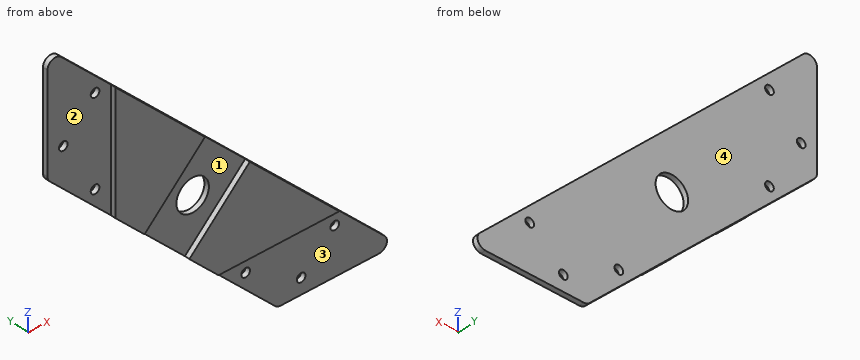
```python
from build123d import *

# Parameters (mm, degrees)
SKETCH1_R           = 10.25
BOSS_EXTRUDE1_DEPTH = 3.175
BOSS_EXTRUDE2_DEPTH = 3.175
FILLET1_R           = 5
CUT_EXTRUDE1_REACH  = 260.624
SKETCH3_R           = 2.75


with BuildPart() as part:
    # Sketch1 → Boss-Extrude1 (new body)
    with BuildSketch(Plane(origin=(0, 0, 0), x_dir=(1, 0, 0), z_dir=(0, 1, 0))):
        Polygon((0, 0), (76.2, 0), (-145, -221.2), (-145, -145), align=None)
        with Locations(Location((-53.45, -91.55, 0), (0, 0, 270))):
            Circle(SKETCH1_R, mode=Mode.SUBTRACT)
    extrude(amount=BOSS_EXTRUDE1_DEPTH)

    # Sketch2 → Boss-Extrude2 (add)
    with BuildSketch(Plane.XZ):
        Polygon((-20.257864376, 96.457864376), (-58.357864376, 58.357864376), (-40, 40), (36.2, 40), align=None)
        Polygon((-105, 105), (-86.642135624, 86.642135624), (-48.542135624, 124.742135624), (-105, 181.2), align=None)
    extrude(amount=BOSS_EXTRUDE2_DEPTH)

    # Fillet1
    fillet1_edges = [part.edges().sort_by_distance(p)[0] for p in [
        (0, 1.5875, 0),
        (76.2, 1.5875, 0),
        (-145, 1.5875, 221.2),
        (-145, 1.5875, 145),
    ]]
    fillet(fillet1_edges, radius=FILLET1_R)

    # Sketch3 → Cut-Extrude1 (cut, up to next)
    with BuildSketch(Plane(origin=(0, 0, 0), x_dir=(-1, 0, 0), z_dir=(0, -1, 0)), mode=Mode.PRIVATE) as cut_extrude1_sk1:
        with Locations(Location((115, -125, 0), (0, 0, 90))):
            Circle(SKETCH3_R)
    cut_extrude1_tool1 = extrude(cut_extrude1_sk1.sketch, amount=-CUT_EXTRUDE1_REACH, mode=Mode.PRIVATE) & part.part
    # Sketch3 → Cut-Extrude1 (cut, up to next)
    with BuildSketch(Plane(origin=(0, 0, 0), x_dir=(-1, 0, 0), z_dir=(0, -1, 0)), mode=Mode.PRIVATE) as cut_extrude1_sk2:
        with Locations(Location((115, -181.2, 0), (0, 0, 90))):
            Circle(SKETCH3_R)
    cut_extrude1_tool2 = extrude(cut_extrude1_sk2.sketch, amount=-CUT_EXTRUDE1_REACH, mode=Mode.PRIVATE) & part.part
    # Sketch3 → Cut-Extrude1 (cut, up to next)
    with BuildSketch(Plane(origin=(0, 0, 0), x_dir=(-1, 0, 0), z_dir=(0, -1, 0)), mode=Mode.PRIVATE) as cut_extrude1_sk3:
        with Locations(Location((135, -160, 0), (0, 0, 90))):
            Circle(SKETCH3_R)
    cut_extrude1_tool3 = extrude(cut_extrude1_sk3.sketch, amount=-CUT_EXTRUDE1_REACH, mode=Mode.PRIVATE) & part.part
    # Sketch3 → Cut-Extrude1 (cut, up to next)
    with BuildSketch(Plane(origin=(0, 0, 0), x_dir=(-1, 0, 0), z_dir=(0, -1, 0)), mode=Mode.PRIVATE) as cut_extrude1_sk4:
        with Locations(Location((-15, -10, 0), (0, 0, 90))):
            Circle(SKETCH3_R)
    cut_extrude1_tool4 = extrude(cut_extrude1_sk4.sketch, amount=-CUT_EXTRUDE1_REACH, mode=Mode.PRIVATE) & part.part
    # Sketch3 → Cut-Extrude1 (cut, up to next)
    with BuildSketch(Plane(origin=(0, 0, 0), x_dir=(-1, 0, 0), z_dir=(0, -1, 0)), mode=Mode.PRIVATE) as cut_extrude1_sk5:
        with Locations(Location((-36.2, -30, 0), (0, 0, 90))):
            Circle(SKETCH3_R)
    cut_extrude1_tool5 = extrude(cut_extrude1_sk5.sketch, amount=-CUT_EXTRUDE1_REACH, mode=Mode.PRIVATE) & part.part
    # Sketch3 → Cut-Extrude1 (cut, up to next)
    with BuildSketch(Plane(origin=(0, 0, 0), x_dir=(-1, 0, 0), z_dir=(0, -1, 0)), mode=Mode.PRIVATE) as cut_extrude1_sk6:
        with Locations(Location((20, -30, 0), (0, 0, 90))):
            Circle(SKETCH3_R)
    cut_extrude1_tool6 = extrude(cut_extrude1_sk6.sketch, amount=-CUT_EXTRUDE1_REACH, mode=Mode.PRIVATE) & part.part
    add(cut_extrude1_tool1.solids().sort_by_distance((-115, 0, 125))[0], mode=Mode.SUBTRACT)
    add(cut_extrude1_tool2.solids().sort_by_distance((-115, 0, 181.2))[0], mode=Mode.SUBTRACT)
    add(cut_extrude1_tool3.solids().sort_by_distance((-135, 0, 160))[0], mode=Mode.SUBTRACT)
    add(cut_extrude1_tool4.solids().sort_by_distance((15, 0, 10))[0], mode=Mode.SUBTRACT)
    add(cut_extrude1_tool5.solids().sort_by_distance((36.2, 0, 30))[0], mode=Mode.SUBTRACT)
    add(cut_extrude1_tool6.solids().sort_by_distance((-20, 0, 30))[0], mode=Mode.SUBTRACT)


solid = part.part
```
Input: part model. Units: mm. Frame: model coordinates. Face numbers are marked on the shaded views. A direction names the side the tool comes from. Coordinates: 2 decimals unless noted, no trailing zeros. Write each loop counter-clockwise with the first axis right and the second up, starting at its lowest first coordinate (ties: lowest second). Pieces come first, ordered by that corner, then holes. Notation, with made-up numbers: (-26, -19) -> (-7, -19) arc R31 ccw to (-7, 10) -> close; hole circle Ø1 at (-13.75, 36.5). An arc over 180 degrees is marked (long way). Answer as a JSON object with one key per item and string values.
1. Access query for the marked faces 3 and 4. Directions: +Z, -Z, +X, -X, +Y, -Y. A direction counts if a zero-diameter tool reaches every point of the face in a straight line with its end or side. Return the directions, or none.
Result set:
{"face 3": "-Z, +X, -X, -Y", "face 4": "+Z, -Z, +X, -X, +Y"}
2. Section A-A on z = 30. Return the cut outline in (x, y) (3 decimals), then the cut area to 3 significant figures.
Result set:
{"outline": "(-30, 0) -> (-22.75, 0) -> (-22.75, 3.175) -> (-30, 3.175) -> close; (-17.25, 0) -> (33.45, 0) -> (33.45, 3.175) -> (-17.25, 3.175) -> close; (38.95, 0) -> (46.2, 0) -> (46.2, 3.175) -> (38.95, 3.175) -> close", "area": "207 mm2"}
3. First-contact query: P1, Ø3.5, axis at y = -1.5, z = 126, coming from the -X side; P2, Ø2.5, axis at x = -2, y = -2, coming from the -Z side; P3, Ø23.5, axis at x = -53.45, z = 91.55, coming from the -Y side. Flat tips, straight axial feed; report the tip coordinate or a pass-through.
Result set:
{"P1": "stops at x = -126.9", "P2": "stops at z = 40", "P3": "stops at y = 0"}
4. Mould query, pull axis X, two halves, no side actions, for the marked faces 1 and 2. Classes: released by +X, released by -X, zero draft, split by the parting line, or undercut.
Result set:
{"face 1": "undercut", "face 2": "zero draft"}
5. Material intervals for line 1 (X direction, y = 2.3, z = 30); line 2 (X direction, y = 2.55, z = 160); line 3 (X direction, y = 2, z = 41.5), sorted ascending. Write a range as from..to.
Result set:
{"line 1": "x = -30..-22.75, -17.25..33.45, 38.95..46.2", "line 2": "x = -145..-137.75, -132.25..-83.8", "line 3": "x = -41.5..34.7"}
6. Section C-C on z = 160. Return the cut outline in (x, y) (3 decimals).
Result set:
{"outline": "(-145, 0) -> (-137.75, 0) -> (-137.75, 3.175) -> (-145, 3.175) -> close; (-132.25, 0) -> (-105, 0) -> (-105, -3.175) -> (-83.8, -3.175) -> (-83.8, 3.175) -> (-132.25, 3.175) -> close"}
7. Section D-D on x = 49. Return the cut outline in (y, z) (3 decimals).
Result set:
{"outline": "(0, 0) -> (3.175, 0) -> (3.175, 27.2) -> (0, 27.2) -> close"}
8. Section B-B on y = -2. Return the cut outline in (x, z), then the cut area to 3 significant figures.
Result set:
{"outline": "(-105, 105) -> (-86.64, 86.64) -> (-48.54, 124.74) -> (-105, 181.2) -> close; (-58.36, 58.36) -> (-40, 40) -> (36.2, 40) -> (-20.26, 96.46) -> close", "area": "5,700 mm2"}
